Work out the finished part from the listing and answer in its coordinate system (mm). Round coordinates to 2 decimals unless told otherwise and drop trailing zeros. Order: outer loops, then holes, each group sorted by start corner. A loop starts at its lowest first (then second) coordinate and runs counter-clockwise, first axis right, second up. Notation, with made-up numbers: M -32,-22 L -16,-22 A31 ccw -16,14 Z; hole C -18.75,47.5 d6. An arc over 180 degrees is marked long. Return JSON: item names as keys, results as strings.
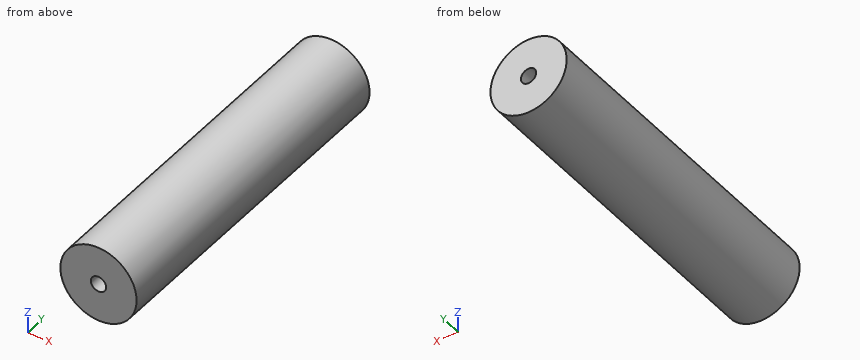
from build123d import *

# Parameters (mm, degrees)
F0_R     = 125
F1_DEPTH = 1100
F2_R     = 25
F3_DEPTH = 50
F4_R     = 25
F5_DEPTH = 50


with BuildPart() as f1:
    # F0 (on Front) → F1 (new body)
    with BuildSketch(Plane.XZ):
        Circle(F0_R)
    extrude(amount=-F1_DEPTH)

    # F2 (on face) → F3 (cut)
    with BuildSketch(Plane.XZ):
        Circle(F2_R)
    extrude(amount=-F3_DEPTH, mode=Mode.SUBTRACT)

    # F4 (on face) → F5 (cut)
    with BuildSketch(Plane(origin=(0, 1100, 0), x_dir=(-1, 0, 0), z_dir=(0, 1, 0))):
        Circle(F4_R)
    extrude(amount=-F5_DEPTH, mode=Mode.SUBTRACT)


solid = f1.part
Item 1: Find section A-A (z = 0). Determine the outline of the cut face in (x, y).
Output:
{"outline": "M -125,0 L -25,0 L -25,50 L 25,50 L 25,0 L 125,0 L 125,1100 L 25,1100 L 25,1050 L -25,1050 L -25,1100 L -125,1100 Z"}
Item 2: Find section D-D (z = 109). Determine the outline of the cut face in (x, y), plus the area to 3 significant figures.
Output:
{"outline": "M -61.19,0 L 61.19,0 L 61.19,1100 L -61.19,1100 Z", "area": "135,000 mm^2"}
Item 3: Find section B-B (x = 0). Determine the outline of the cut face in (y, z).
Output:
{"outline": "M 0,-125 L 1100,-125 L 1100,-25 L 1050,-25 L 1050,25 L 1100,25 L 1100,125 L 0,125 L 0,25 L 50,25 L 50,-25 L 0,-25 Z"}
Item 4: Each of these flat-tipped pins is pushed along its axis until it touches: pin 1 (1.5 mm diameter, centred on y = 810.5, z = 75.5, fed in from -X); pin 2 (3 mm diameter, centred on x = 18.5, y = 447, fed in from +Z); pin 3 (4 mm diameter, centred on x = -49, y = 643, fed in from +Z). Where does it stop, or does it pass through?
Output:
{"pin 1": "stops at x = -100.19", "pin 2": "stops at z = 123.84", "pin 3": "stops at z = 115.83"}
Item 5: Find section C-C (y = 956.5). Determine the outline of the cut face in (x, z).
Output:
{"outline": "C 0,0 d250"}
Item 6: Consider line 1 along Z through (x, y) = (0, 14); line 2 along X through (y, z) = (85, 46.5); line 3 along Z through (x, y) = (81, 890). Determine where each line is inside the solid, lowest interval first. Write a range as [from, to].
Output:
{"line 1": "z = [-125, -25], [25, 125]", "line 2": "x = [-116.03, 116.03]", "line 3": "z = [-95.21, 95.21]"}
